Model file for the job. Use its own axes, mm. A direction names the side the tool comes from. Round coordinates to 2 decimals unless told otherwise and drop trailing zeros. Write each loop counter-clockwise with the first axis right and the second up, starting at its lowest first coordinate (ties: lowest second). Pieces come first, ordered by that corner, then holes. Notation, with made-up numbers: (49, 67) - (64, 67) arc R8 cw to (64, 73) - close; hole circle Ø10 at (-23, -5). An arc over 180 degrees is marked (long way). One line per item, written item: value.
from build123d import *

# Parameters (mm, degrees)
PAD_DEPTH = 9.5


with BuildPart() as part:
    # Sketch → Pad (new body)
    with BuildSketch(Plane.XY):
        Polygon((-41.25, 27.25), (-29.1, 27.25), (-29.3, 26.05), (-25.7, 26.05), (-25.9, 27.25), (25.9, 27.25), (25.7, 26.05), (29.3, 26.05), (29.1, 27.25), (41.25, 27.25), (41.25, 24.35), (42.85, 24.6), (42.85, 20.4), (41.25, 20.65), (41.25, 1.85), (42.85, 2.1), (42.85, -2.1), (41.25, -1.85), (41.25, -20.65), (42.85, -20.4), (42.85, -24.6), (41.25, -24.35), (41.25, -27.25), (29.35, -27.25), (29.6, -28.85), (25.4, -28.85), (25.65, -27.25), (-25.65, -27.25), (-25.4, -28.85), (-29.6, -28.85), (-29.35, -27.25), (-41.25, -27.25), (-41.25, -24.1), (-40.05, -24.3), (-40.05, -20.7), (-41.25, -20.9), (-41.25, -1.6), (-40.05, -1.8), (-40.05, 1.8), (-41.25, 1.6), (-41.25, 20.9), (-40.05, 20.7), (-40.05, 24.3), (-41.25, 24.1), align=None)
    extrude(amount=-PAD_DEPTH)


solid = part.part
1. Band-saw the part on A-A on x = -28. Write the cut outline in (y, z).
Report:
outline: (-28.85, -9.5) - (26.05, -9.5) - (26.05, 0) - (-28.85, 0) - close
2. Wall check: probe 1 along X at (y, z) = (-6, -6.5); probe 2 along Y at (x, z) = (5.5, -4); probe 3 along X at (y, z) = (-1.5, -4.25). Give the ranges that are in metal, low to high. Write a range as [from, to].
Report:
probe 1: [-41.25, 41.25]
probe 2: [-27.25, 27.25]
probe 3: [-40.05, 42.85]
3. Band-saw the part on B-B on y = 3.5. Write the cut outline in (x, z).
Report:
outline: (-41.25, -9.5) - (41.25, -9.5) - (41.25, 0) - (-41.25, 0) - close
4. Tool access for faces 1 (the face through (-25.527, -28.039, -4.684)), 2 (the face through (29.473, -28.039, -4.684)), 3 (the face through (1, 0, -9.5)): list every direction of +Z, -Z, +X, -X, +Y, -Y with a clear straight run to the whole face (end or side of a thin tool).
Report:
face 1: +Z, -Z
face 2: +Z, -Z, +X
face 3: -Z, +X, -X, +Y, -Y
5. Drop flat-ended pins along their axis: pin 1 (5 mm diameter, centred on x = -8, z = -6, fed in from -Y); pin 2 (2 mm diameter, centred on y = 18.5, z = -8, fed in from +X); pin 3 (1.1 mm diameter, centred on x = -28, z = -2.5, fed in from +Y); pin 4 (4 mm diameter, centred on y = 22.5, z = -4, fed in from -X). Give the stop position or say it passes through.
Report:
pin 1: y = -27.25
pin 2: x = 41.25
pin 3: y = 26.05
pin 4: x = -41.25
6. Mould opens along Y. For faces 4 (the face through (-29.477, -28.061, -4.684)), 5 (the face through (-40.05, 0, -5)), 6 (the face through (-41.25, -11, -5)), 7 (the face through (42.039, 24.473, -4.684)) say: released by +Y, released by -Y, zero draft, split by the parting line, or undercut.
Report:
face 4: undercut
face 5: undercut
face 6: zero draft
face 7: released by +Y
